Part print with two shaded views. Sizes in mm from the minimum x, y, z corner. Round coordinates to 2 decimals unless told otherwise and drop trailing zeros. Loops run counter-clockwise (first coordinate to the right, second up) from the corner with the lowest first, then second, coordinate; pieces in that order, holes last.
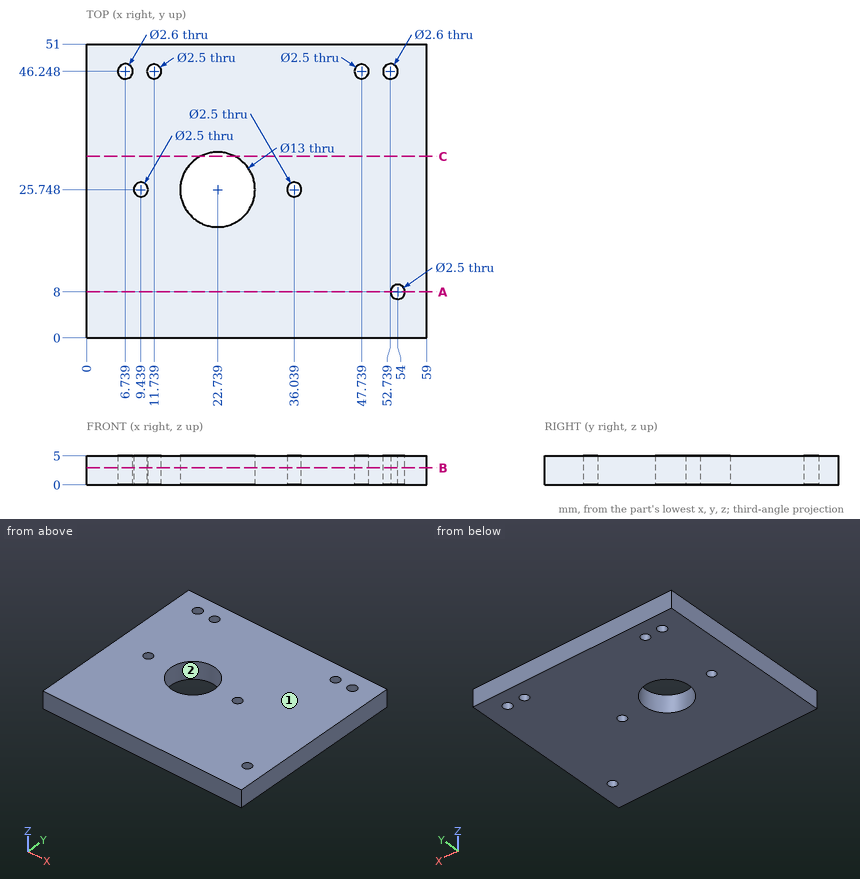
Item 1: Cut at A-A (y = 8). List the corners of the cut face in (x, z).
Verdict:
outline: (0, 0) - (52.75, 0) - (52.75, 5) - (0, 5) - close; (55.25, 0) - (59, 0) - (59, 5) - (55.25, 5) - close
Item 2: Wall check: L1, parallel to Y at x = 21, z = 1.35 (1 decimal); L2, parallel to Y at x = 12, z = 2.9 (1 decimal); L3, parallel to X at y = 30, z = 4.6 (1 decimal). Give the ranges that are in metal, low to high.
Verdict:
L1: y = 0 to 19.5, 32 to 51
L2: y = 0 to 45, 47.5 to 51
L3: x = 0 to 17.8, 27.7 to 59
Item 3: Cut at C-C (y = 31.5). List the corners of the cut face in (x, z) (1 decimal), plus the area to 3 significant figures.
Verdict:
outline: (0, 0) - (19.7, 0) - (19.7, 5) - (0, 5) - close; (25.8, 0) - (59, 0) - (59, 5) - (25.8, 5) - close
area: 265 mm2
Item 4: Cut at B-B (z = 2.95). State how many separate pieces and enclosed holes the cut face has, plus the area to 3 significant figures.
Verdict:
separate pieces: 1
enclosed holes: 8
area: 2,840 mm2
Item 5: Mould opens along Y. For the marked faces 1 and 2 say: released by +Y, released by -Y, zero draft, split by the parting line, or undercut.
Verdict:
face 1: zero draft
face 2: undercut
